Autodesk Inventor part; units mm, degrees
ref_plane "YZ Plane" through (0, 0, 0) normal (1, 0, 0) x (0, 1, 0)
ref_plane "XZ Plane" through (0, 0, 0) normal (0, 1, 0) x (-1, 0, 0)
ref_plane "XY Plane" through (0, 0, 0) normal (0, 0, 1) x (1, 0, 0)
sketch "Skizze1" plane through (0, 0, 0) normal (1, 0, 0) x (0, 1, 0)
  line L0 (-20, -20) -> (20, -20)
  line L1 (20, -20) -> (20, 20)
  line L2 (20, 20) -> (-20, 20)
  line L3 (-20, 20) -> (-20, -20)
  line L4 (-20, -20) -> (20, 20) construction
  line L5 (20, -20) -> (-20, 20) construction
  line L6 (-16, -16) -> (16, -16) construction
  line L7 (16, -16) -> (16, 16) construction
  line L8 (16, 16) -> (-16, 16) construction
  line L9 (-16, 16) -> (-16, -16) construction
  line L10 (-16, -16) -> (16, 16) construction
  line L11 (16, -16) -> (-16, 16) construction
  circle A0 centre (16, 16) radius 2.25
  circle A1 centre (16, -16) radius 2.25
  circle A2 centre (-16, -16) radius 2.25
  circle A3 centre (-16, 16) radius 2.25
  line L12 (-20, 20) -> (-32, 20)
  line L13 (-32, 20) -> (-32, -20)
  line L14 (-32, -20) -> (-20, -20)
  line L15 (-20, -20) -> (-20, 20)
  point P0 (0, 0)
  dimension "d0" = 40
  dimension "d1" = 40
  dimension "d2" = 32
  dimension "d3" = 32
  dimension "d4" = 4.5
  dimension "d5" = 4.5
  dimension "d6" = 4.5
  dimension "d7" = 4.5
  dimension "d8" = 12
extrude "Extrusion1" add sketch "Skizze1" along normal blind 6
ref_plane "Arbeitsebene1" through (0, -32, 20) normal (0, 0, 1) x (1, 0, 0)
sketch "Skizze2" plane through (0, -32, 20) normal (0, 0, 1) x (1, 0, 0)
  line L0 (0, 52) -> (0, 0)
  line L1 (0, 0) -> (6, 0)
  line L2 (6, 52) -> (6, 0)
  line L3 (0, 52) -> (6, 52)
  line L4 (-20, 6) -> (-14, 6)
  line L5 (-14, 6) -> (-14, -39)
  line L6 (-14, -39) -> (-20, -39)
  line L7 (-20, -39) -> (-20, 6)
  line L8 (0, 0) -> (-14, -4)
  line L9 (-14, 6) -> (0, 6)
  point P0 (0, 32)
  point P1 (-17, -39)
  point P2 (-17, 6)
  dimension "d12" = 6
  dimension "d13" = 45
  dimension "d14" = 6
  dimension "d15" = 14
  dimension "d16" = 10
extrude "Extrusion2" add sketch "Skizze2" against normal up to surface (40 mm away) contours L0 L8 L5 L9 | L5 L6 L7 L4
chamfer "Fasen1" distance 4 angle 45 6 edges at (-20, -26, 0) (0, -26, 0) (-17, -71, -20) (-17, -71, 20) (3, 20, -20) (3, 20, 20)
sketch "Skizze3" plane through (-14, -36, 20) normal (1, 0, 0) x (0, 0, -1)
  line L0 (4, -35) -> (0, -31)
  line L1 (4, -35) -> (36, -35)
  line L2 (40, -31) -> (36, -35)
  line L3 (40, 0) -> (40, -31)
  line L4 (0, 0) -> (40, 0)
  line L5 (0, -31) -> (0, 0)
  circle A0 centre (20, -15) radius 20
  circle A1 centre (20, -15) radius 17.5
  point P0 (20, 36)
  dimension "d22" = 35
extrude "Extrusion3" cut sketch "Skizze3" along normal through all contours A1 L4 | L4 A1
sketch "Skizze4" plane through (-14, -67, 20) normal (1, 0, 0) x (0, 0, -1)
  line L0 (0, 31) -> (10.9861, 31)
  line L1 (0, 0) -> (0, 31)
  line L2 (4, -4) -> (0, 0)
  line L3 (4, -4) -> (36, -4)
  line L4 (40, 0) -> (36, -4)
  line L5 (40, 31) -> (40, 0)
  line L6 (29.0139, 31) -> (40, 31)
  arc A0 (29.0139, 31) -> (10.9861, 31) centre (20, 16) ccw
  circle A1 centre (20, 16) radius 17.5
  circle A2 centre (2.5, 16) radius 2
  circle A3 centre (37.5, 16) radius 2
  point P0 (20, 67)
  dimension "d25" = 4
  dimension "d26" = 4
extrude "Extrusion4" cut sketch "Skizze4" against normal blind 10 contours A2 A1 | A1 A2 | A3 A1 | A1 A3
sketch "Skizze5" plane through (-14, -67, 20) normal (1, 0, 0) x (0, 0, -1)
  arc A0 (29.0139, 31) -> (10.9861, 31) centre (20, 16) ccw
  line L0 (0, 35) -> (40, 35)
  line L1 (0, 31) -> (0, 35)
  line L2 (0, 31) -> (10.9861, 31)
  circle A1 centre (20, 16) radius 11
  line L3 (29.0139, 31) -> (40, 31)
  line L4 (40, 35) -> (40, 31)
  point P0 (20, 67)
  dimension "d29" = 22
extrude "Extrusion5" cut sketch "Skizze5" against normal blind 10 contours A1
properties part number "40_XYZstage_micrometer_motorized_nema8_samplemount_lightsheet_screwed"
Here's how the part is built. I have some questions about the finished solid (model axes, mm). A direction names the side the tool comes from. Give positions to 0.01 mm unless a question says otherwise; leave off trailing zeros. Loops run counter-clockwise (first coordinate to the right, second up) from the corner with the lowest first, then second, coordinate; pieces in that order, holes last. Notation, with made-up numbers: M -22,33.5 L 21,33.5 A8 ccw 21,40.5 Z; hole C -31.5,67.25 d7. An arc over 180 degrees is marked long. Return JSON: item names as keys, results as strings.
Item 1: Imagine slicing it at B-B on y = -16. List the corners of the cut face in (x, z) for me, then the cut area to 3 significant figures.
A:
{"outline": "M 0,-20 L 6,-20 L 6,-18.25 L 0,-18.25 Z; M 0,-13.75 L 6,-13.75 L 6,13.75 L 0,13.75 Z; M 0,18.25 L 6,18.25 L 6,20 L 0,20 Z", "area": "186 mm^2"}
Item 2: Please list where these lines run through material, in increasing order: line 1 (Z direction, x = 3.4, y = 16); line 2 (X direction, y = -41.5, z = -13.5); line 3 (X direction, y = 4, z = 8).
A:
{"line 1": "z = -20 to -18.25, -13.75 to 13.75, 18.25 to 20", "line 2": "x = -20 to -14", "line 3": "x = 0 to 6"}
Item 3: Imagine slicing it at C-C on x = -17.5. List the corners of the cut face in (y, z) for me.
A:
{"outline": "M -71,-16 L -67,-20 L -27.5,-20 L -27.5,20 L -67,20 L -71,16 Z; hole C -51,0 d22; hole C -51,-17.5 d4; hole C -51,17.5 d4"}
Item 4: Imagine slicing it at A-A on z = 0. List the corners of the cut face in (x, y) for me, then the cut area to 3 significant figures.
A:
{"outline": "M -20,-71 L -14,-71 L -14,-62 L -20,-62 Z; M -20,-40 L -14,-40 L -14,-33.5 L -5.25,-33.5 L 0,-32 L 6,-32 L 6,20 L 0,20 L 0,-22 L -4,-26 L -16,-26 L -20,-30 Z", "area": "551 mm^2"}
Item 5: Imagine slicing it at D-D on x = 1.5. List the corners of the cut face in (y, z) for me.
A:
{"outline": "M -32,-20 L 16,-20 L 20,-16 L 20,16 L 16,20 L -32,20 Z; hole C -16,-16 d4.5; hole C -16,16 d4.5; hole C 16,-16 d4.5; hole C 16,16 d4.5"}
Item 6: Thinking about a two-plate mould opening in Z: for faces 3 (the cylindrical face through (2.958, -14.962, -14.004)), 4 (the flat face through (-17, -69, -18)), 5 (the flat face through (3, -32, 0)), which applies, released by +Z, released by -Z, zero draft, split by the parting line, or undercut?
A:
{"face 3": "undercut", "face 4": "released by -Z", "face 5": "zero draft"}
Item 7: On a 3-axis mill with a long thin cutter (end or side, diameter ignored), from which of +Z, -Z, +X, -X, +Y, -Y can I reach the whole of each face in a straight line? I mean faces 1 (the flat face through (3, 18, -18)), 2 (the flat face through (-10, -26, 0)). Say none if no direction works.
A:
{"face 1": "-Z, +X, -X, +Y", "face 2": "+Z, -Z, -X, +Y"}
Item 8: I'm going to push flat-ended pins straight in: pin 1 Ø1.8 at (x, z) = (3, 8.5) entering from -Y; pin 2 Ø3 at (x, z) = (-5, -15.5) entering from +Y; pin 3 Ø13 at (x, z) = (-12.5, 3.5) entering from +Y. Where does each tip first touch, or does it pass through?
A:
{"pin 1": "stops at y = -32", "pin 2": "stops at y = -25.5", "pin 3": "stops at y = -26"}
